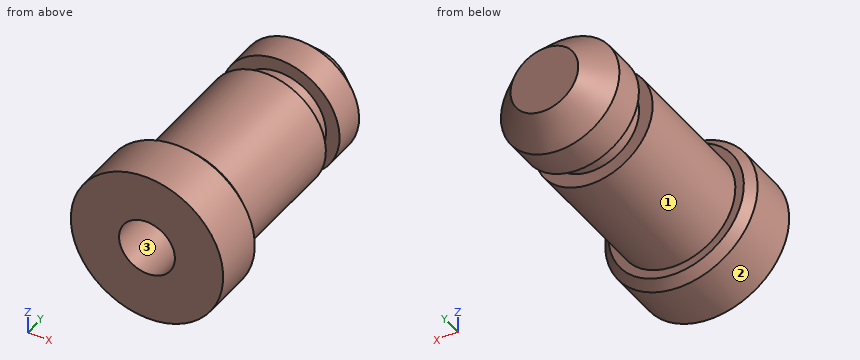
from build123d import *

# Parameters (mm, degrees)
SKETCH_1_R             = 3.5
EXTRUDE_1_DEPTH        = 8
SKETCH_2_W             = 1
SKETCH_2_H             = 3.5
HOLE_WIZARD_M4_1_D     = 3.3
HOLE_WIZARD_M4_1_DEPTH = 10.1
HOLE_WIZARD_M4_1_TIP   = 0.991420021
CHAMFER_1_SIZE         = 1.5
SKETCH_6_W             = 0.8
SKETCH_6_H             = 1.3
CHAMFER_2_SIZE         = 0.5


with BuildPart() as part:
    # 草图1 → 凸台-拉伸1 (new, symmetric)
    with BuildSketch(Plane(origin=(0, 0, 0), x_dir=(1, 0, 0), z_dir=(0, 1, 0))):
        with Locations(Location((0, 0, 0), (0, 0, 270))):
            Circle(SKETCH_1_R)
    extrude(amount=EXTRUDE_1_DEPTH, both=True)

    # 草图2 → 旋转1 (revolve)
    with BuildSketch(Plane.XY, mode=Mode.PRIVATE) as revolve_1_sk:
        with Locations((4, -6.25)):
            Rectangle(SKETCH_2_W, SKETCH_2_H)
    revolve(revolve_1_sk.sketch.rotate(Axis((0, 8, 0), (0, -1, 0)), 270), axis=Axis((0, 8, 0), (0, -1, 0)))

    # M4 螺纹孔1
    with Locations(Plane(origin=(0, -8, 0), x_dir=(-1, 0, 0), z_dir=(0, -1, 0))):
        with Locations((0, 0)):
            Hole(HOLE_WIZARD_M4_1_D / 2, depth=HOLE_WIZARD_M4_1_DEPTH)
            with Locations((0, 0, -(HOLE_WIZARD_M4_1_DEPTH + HOLE_WIZARD_M4_1_TIP / 2))):  # 118° drill point
                Cone(0, HOLE_WIZARD_M4_1_D / 2, HOLE_WIZARD_M4_1_TIP, mode=Mode.SUBTRACT)

    # 倒角1
    chamfer_1_edges = [part.edges().sort_by_distance(p)[0] for p in [
        (0, 8, -3.5),
    ]]
    chamfer(chamfer_1_edges, length=CHAMFER_1_SIZE)

    # 草图6 → 切除-旋转1 (revolve, cut)
    with BuildSketch(Plane.XY, mode=Mode.PRIVATE) as cut_revolve_1_sk:
        with Locations((3.1, 4)):
            Rectangle(SKETCH_6_W, SKETCH_6_H)
    revolve(cut_revolve_1_sk.sketch.rotate(Axis((0, 8, 0), (0, -1, 0)), 270), axis=Axis((0, 8, 0), (0, -1, 0)), mode=Mode.SUBTRACT)

    # 倒角2
    chamfer_2_edges = [part.edges().sort_by_distance(p)[0] for p in [
        (0, -4.5, 4.5),
    ]]
    chamfer(chamfer_2_edges, length=CHAMFER_2_SIZE)


solid = part.part
Model file for the job. Use its own axes, mm. Face numbers are marked on the shaded views. A direction names the side the tool comes from. Give positions to 0.01 mm unless a question says otherwise; leave off trailing zeros.
1) Flat gauge pins, fed straight in: pin 1 Ø2 at (x, z) = (1.5, 0.5) entering from -Y; pin 2 Ø1 at (x, z) = (-0.5, -3.5) entering from +Y; pin 3 Ø1 at (y, z) = (-3, 0) entering from +X. Where does each tip first touch, or does it go through?
2) Wall check: line 1 (Y direction, x = 0.75, z = -3.5); line 2 (Y direction, x = -2.5, z = -1.5); line 3 (Z direction, x = 1.25, y = 0). Give the ranges that are in metal, low to high.
3) Tool access for the marked faces 1, 2 and 3: list every direction of +Z, -Z, +X, -X, +Y, -Y with a clear straight run to the whole face (end or side of a thin tool).
Answer block:
1. pin 1: stops at y = -8
1. pin 2: stops at y = 6.96
1. pin 3: stops at x = 3.5
2. line 1: y = -8 to -4.5
2. line 2: y = -8 to 3.35, 4.65 to 7.08
2. line 3: z = -3.27 to -1.08, 1.08 to 3.27
3. face 1: +Y
3. face 2: +Y, -Y
3. face 3: -Y
